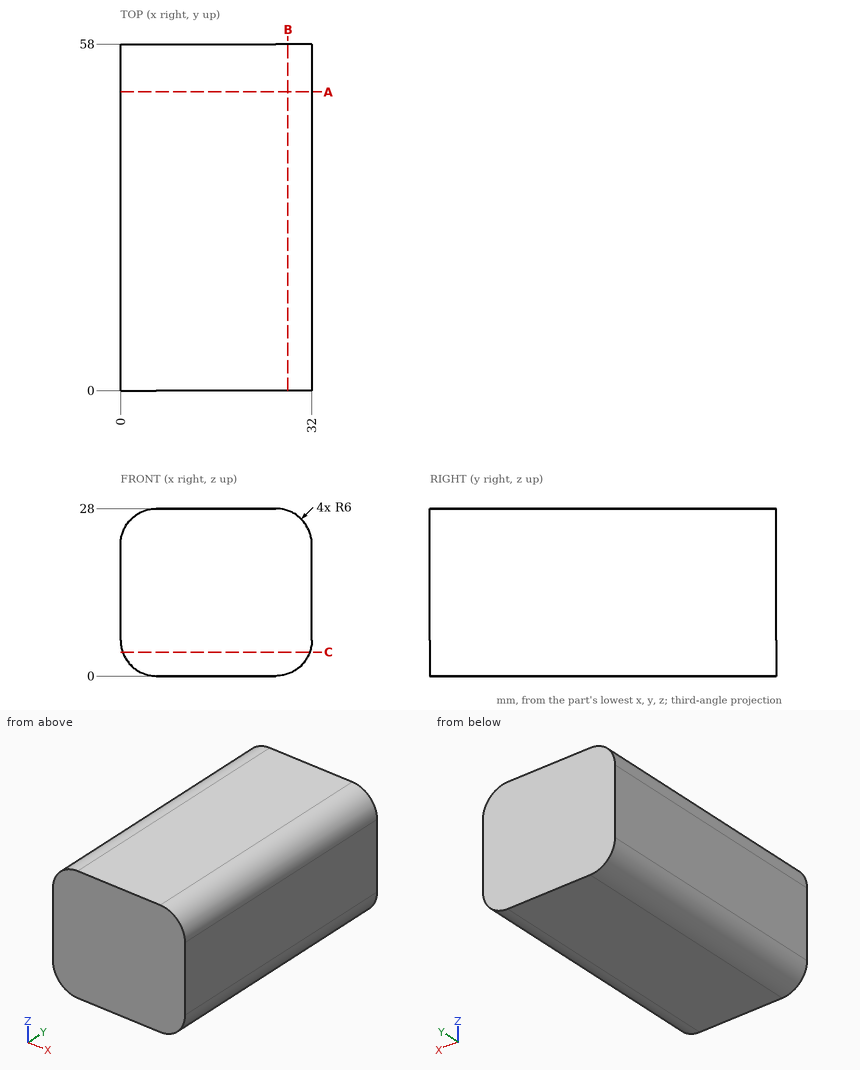
Job drawing, mm, ordinate dimensions from the low corner. One solid piece. Coordinates: 2 decimals unless noted, no trailing zeros. Order: outer loops, then holes, each group sorted by start corner. A loop starts at its lowest first (then second) coordinate and runs counter-clockwise, first axis right, second up. Notation, with made-up numbers: (50, 30.5) -> (62, 30.5) arc R19 ccw to (62, 53.5) -> close; hole circle Ø11 at (7.25, -13.75). An arc over 180 degrees is marked (long way). Answer in a Markdown table with one row per item. Add a question column.
Q1. Band-saw the part on B-B, the plane x = 28. List the corners of the cut face in (y, z).
Q2. Band-saw the part on C-C, the plane z = 4. List the corners of the cut face in (x, y).
Q3. Band-saw the part on A-A, the plane y = 50. List the corners of the cut face in (x, z).
Q4. Wall check: line 1 along X through (y, z) = (45.5, 1.5); line 2 along Z through (x, y) = (3, 40.5); line 3 along X through (y, z) = (48.5, 3.75). Give the ranges that are in metal, low to high. Write a range as [from, to].
Answers follow:
| question | item | result |
|---|---|---|
| 1 | outline | (0, 0.34) -> (58, 0.34) -> (58, 27.66) -> (0, 27.66) -> close |
| 2 | outline | (0.34, 0) -> (31.66, 0) -> (31.66, 58) -> (0.34, 58) -> close |
| 3 | outline | (0, 6) arc R6 ccw to (6, 0) -> (26, 0) arc R6 ccw to (32, 6) -> (32, 22) arc R6 ccw to (26, 28) -> (6, 28) arc R6 ccw to (0, 22) -> close |
| 4 | line 1 | [2.03, 29.97] |
| 4 | line 2 | [0.8, 27.2] |
| 4 | line 3 | [0.44, 31.56] |
